Could you check a few things on this model? Use its own coordinates, in mm. Round coordinates to 2 decimals unless told otherwise and drop trailing zeros. Loops run counter-clockwise (first coordinate to the right, second up) from the corner with the lowest first, then second, coordinate; pieces in that order, holes last. Notation, with made-up numbers: (70.5, 68) -> (98.5, 68) arc R8 ccw to (98.5, 73) -> close; hole circle Ø1 at (80, -25.5). An arc over 180 degrees is marked (long way). One line per item, written item: value.
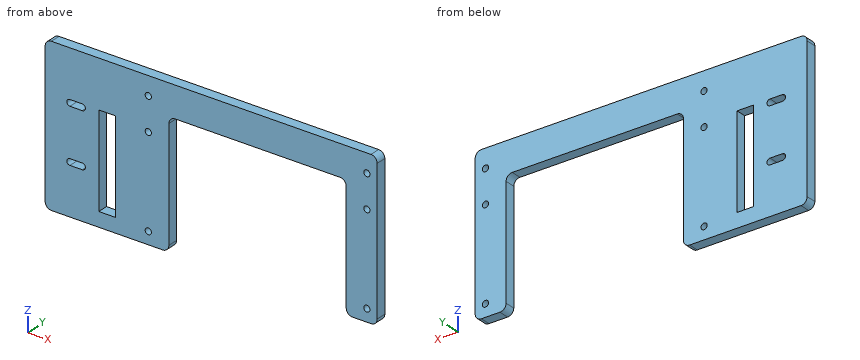
```python
from build123d import *

# Parameters (mm, degrees)
SKETCH_1_R          = 1.5
EXTRUDE_1_DEPTH     = 5
SKETCH_11_W         = 8
SKETCH_11_H         = 45
CUT_EXTRUDE_6_DEPTH = 118.584012519
FILLET_1_R          = 3
CUT_EXTRUDE_7_DEPTH = 118.584012519


with BuildPart() as part:
    # 草图1 → 凸台-拉伸1 (new body)
    with BuildSketch(Plane(origin=(0, 0, 0), x_dir=(1, 0, 0), z_dir=(0, 1, 0))):
        Polygon((0, 0), (0, 60), (-60, 60), (-60, -15), (101, -15), (101, 60), (86, 60), (86, 0), align=None)
        with Locations(Location((-10, 54, 0), (0, 0, 270))):
            Circle(SKETCH_1_R, mode=Mode.SUBTRACT)
        with Locations(Location((-10, -6, 0), (0, 0, 90))):
            Circle(SKETCH_1_R, mode=Mode.SUBTRACT)
        with Locations(Location((96, 54, 0), (0, 0, 270))):
            Circle(SKETCH_1_R, mode=Mode.SUBTRACT)
        with Locations(Location((96, -6, 0), (0, 0, 270))):
            Circle(SKETCH_1_R, mode=Mode.SUBTRACT)
        with Locations(Location((96, 10, 0), (0, 0, 270))):
            Circle(SKETCH_1_R, mode=Mode.SUBTRACT)
        with Locations(Location((-10, 10, 0), (0, 0, 90))):
            Circle(SKETCH_1_R, mode=Mode.SUBTRACT)
    extrude(amount=EXTRUDE_1_DEPTH)

    # 草图11 → 切除-拉伸6 (cut, through all)
    with BuildSketch(Plane(origin=(0, 5, 0), x_dir=(1, 0, 0), z_dir=(0, 1, 0))):
        with Locations((-30, 30.5)):
            Rectangle(SKETCH_11_W, SKETCH_11_H)
    extrude(amount=-CUT_EXTRUDE_6_DEPTH, mode=Mode.SUBTRACT)

    # 圆角1
    fillet_1_edges = [part.edges().sort_by_distance(p)[0] for p in [
        (86, 2.5, 0),
        (86, 2.5, -60),
        (101, 2.5, -60),
        (101, 2.5, 15),
        (-60, 2.5, 15),
        (-60, 2.5, -60),
        (0, 2.5, -60),
        (0, 2.5, 0),
    ]]
    fillet(fillet_1_edges, radius=FILLET_1_R)

    # 草图12 → 切除-拉伸7 (cut, through all)
    with BuildSketch(Plane(origin=(0, 5, 0), x_dir=(1, 0, 0), z_dir=(0, 1, 0))):
        with BuildLine():
            Line((-48, 37.1), (-42, 37.1))
            ThreePointArc((-42, 37.1), (-40.5, 35.6), (-42, 34.1))
            Line((-42, 34.1), (-48, 34.1))
            ThreePointArc((-48, 34.1), (-49.5, 35.6), (-48, 37.1))
        make_face()
        with BuildLine():
            Line((-48, 7.9), (-42, 7.9))
            ThreePointArc((-42, 7.9), (-40.5, 9.4), (-42, 10.9))
            Line((-42, 10.9), (-48, 10.9))
            ThreePointArc((-48, 10.9), (-49.5, 9.4), (-48, 7.9))
        make_face()
    extrude(amount=-CUT_EXTRUDE_7_DEPTH, mode=Mode.SUBTRACT)


solid = part.part
```
(1) For pin 1 Ø5 at (x, z) = (-10, -54) entering from -Y, with a flat end and sliding along its axis, tell me the tip position at first contact or that it passes through.
Results below:
pin 1: stops at y = 0
(2) Imagine slicing it at C-C on y = 2.3. Give the number of separate pieces and of enclosed holes in the cut face, then the cut area to 3 significant figures.
Results below:
separate pieces: 1
enclosed holes: 9
area: 6,450 mm²
(3) Imagine slicing it at D-D on x = -10. Write out the boundary of the cut face in (y, z).
Results below:
outline: (0, -60) -> (5, -60) -> (5, -55.5) -> (0, -55.5) -> close; (0, -52.5) -> (5, -52.5) -> (5, -11.5) -> (0, -11.5) -> close; (0, -8.5) -> (5, -8.5) -> (5, 4.5) -> (0, 4.5) -> close; (0, 7.5) -> (5, 7.5) -> (5, 15) -> (0, 15) -> close
(4) Please list where these lines run through material, in increasing order: L1, parallel to Z at x = 96, y = 3.8; L2, parallel to X at y = 3.95, z = -25; L3, parallel to X at y = 1.45, z = 6.
Results below:
L1: z = -60 to -55.5, -52.5 to -11.5, -8.5 to 4.5, 7.5 to 15
L2: x = -60 to -34, -26 to 0, 86 to 101
L3: x = -60 to -11.5, -8.5 to 94.5, 97.5 to 101
(5) Imagine slicing it at B-B on z = 6. Write out the boundary of the cut face in (x, y).
Results below:
outline: (-60, 0) -> (-11.5, 0) -> (-11.5, 5) -> (-60, 5) -> close; (-8.5, 0) -> (94.5, 0) -> (94.5, 5) -> (-8.5, 5) -> close; (97.5, 0) -> (101, 0) -> (101, 5) -> (97.5, 5) -> close
(6) Imagine slicing it at A-A on x = -30. Write out the boundary of the cut face in (y, z).
Results below:
outline: (0, -60) -> (5, -60) -> (5, -53) -> (0, -53) -> close; (0, -8) -> (5, -8) -> (5, 15) -> (0, 15) -> close
